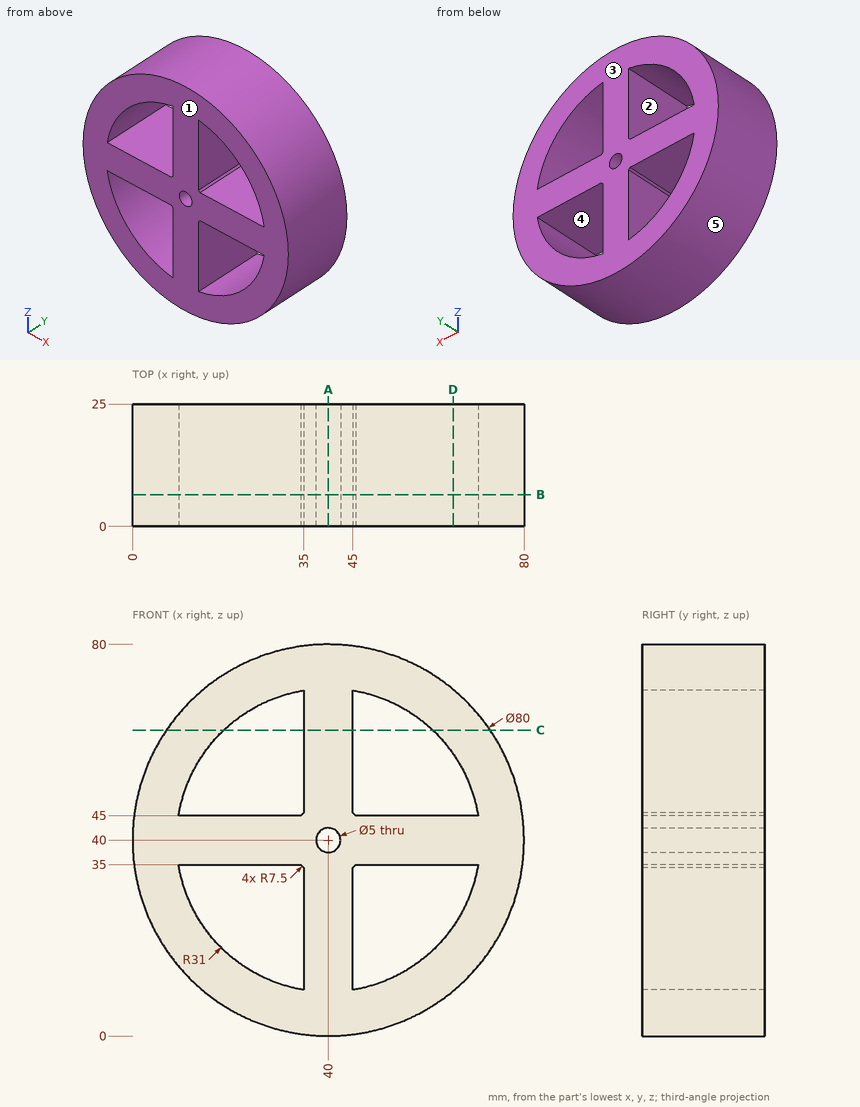
Can you work these out from the drawing? Everything is in mm from the part's minimum corner. A direction names the side the tool comes from. Coordinates: 2 decimals unless noted, no trailing zeros. Loops run counter-clockwise (first coordinate to the right, second up) from the corner with the lowest first, then second, coordinate; pieces in that order, holes last.
1. If we mould it in two halves opening along Z, with no side actions, what happens to the marked faces 3, 4 and 5? For each: pulls with the +Z half, pulls with the -Z half, needs draft (parallel to the pull), parting line crosses it, or undercut.
2. Imagine slicing it at A-A, the plane x = 40. Please give me the cut outline in (y, z), and give its area (4 significant figures).
3. For P1, Ø6, axis at y = 18, z = 12, coming from the +X side (3 decimals); P2, Ø8, axis at x = 50, y = 3.5, coming from the +Z side; P3, Ø12, axis at y = 11.5, z = 20, coming from the -X side; P4, Ø2, axis at x = 20, z = 67.5, coming from the -Y side, each with a flat end and sliding along its axis, tell me the tip position at first contact or that it passes through.
4. Imagine slicing it at B-B, the plane y = 6.5. Please give me the cut outline in (x, z).
5. Imagine slicing it at D-D, the plane x = 65.5. Please give me the cut outline in (y, z).
6. For the marked faces 1 and 2, which set-ups out of +Z, -Z, +X, -X, +Y, -Y let a thin tool reach every point of the face, with its end or its side?
7. Imagine slicing it at C-C, the plane z = 62.5. Please give me the cut outline in (x, y) (3 decimals).
8. I need wall thicknesses on L1, parallel to X at y = 4.25, z = 68.5; L2, parallel to Z at x = 13, y = 12.75; L3, parallel to Z at x = 48.5, y = 21.5. Which ranges of each line are inside material? Lowest first, please.
Taken from the geometry:
1. face 3: needs draft
1. face 4: undercut
1. face 5: parting line crosses it
2. outline: (0, 0) - (25, 0) - (25, 37.5) - (0, 37.5) - close; (0, 42.5) - (25, 42.5) - (25, 80) - (0, 80) - close
2. area: 1,875 mm2
3. P1: stops at x = 71.225
3. P2: stops at z = 79.55
3. P3: stops at x = 2.53
3. P4: stops at y = 0
4. outline: circle Ø80 at (40, 40); hole (9.41, 35) arc R31 ccw to (35, 9.41) - (35, 34.41) arc R7.5 cw to (34.41, 35) - close; hole (9.41, 45) - (34.41, 45) arc R7.5 cw to (35, 45.59) - (35, 70.59) arc R31 ccw to start; hole circle Ø5 at (40, 40); hole (45, 9.41) arc R31 ccw to (70.59, 35) - (45.59, 35) arc R7.5 cw to (45, 34.41) - close; hole (45, 45.59) arc R7.5 cw to (45.59, 45) - (70.59, 45) arc R31 ccw to (45, 70.59) - close
5. outline: (0, 9.18) - (25, 9.18) - (25, 22.37) - (0, 22.37) - close; (0, 35) - (25, 35) - (25, 45) - (0, 45) - close; (0, 57.63) - (25, 57.63) - (25, 70.82) - (0, 70.82) - close
6. face 1: +Z, -Z, +X, -X, -Y
6. face 2: +Y, -Y
7. outline: (6.928, 0) - (18.675, 0) - (18.675, 25) - (6.928, 25) - close; (35, 0) - (45, 0) - (45, 25) - (35, 25) - close; (61.325, 0) - (73.072, 0) - (73.072, 25) - (61.325, 25) - close
8. L1: x = 11.93 to 27.8, 35 to 45, 52.2 to 68.07
8. L2: z = 10.49 to 24.77, 35 to 45, 55.23 to 69.51
8. L3: z = 0.91 to 10.19, 35 to 45, 69.81 to 79.09
